```python
from build123d import *

# Parameters (mm, degrees)
BOSS_EXTRUDE1_DEPTH = 40
CUT_EXTRUDE1_REACH  = 53.556
SKETCH2_R           = 2.5
CUT_EXTRUDE2_REACH  = 53.556
SKETCH3_R           = 2.5
SKETCH4_W           = 70
SKETCH4_H           = 70
BOSS_EXTRUDE2_DEPTH = 3
SKETCH8_W           = 54
SKETCH8_H           = 54
SKETCH8_W_2         = 50
SKETCH8_H_2         = 50
CUT_EXTRUDE7_DEPTH  = 0.5
CUT_EXTRUDE8_REACH  = 112.467
SKETCH9_R           = 1.55
CUT_EXTRUDE9_REACH  = 112.467
SKETCH10_W          = 40
SKETCH10_H          = 20
FILLET1_R           = 5


with BuildPart() as part:
    # Sketch1 → Boss-Extrude1 (new body)
    with BuildSketch(Plane.XY):
        Polygon((0, 0), (0, 23), (23, 23), (23, 20), (3, 20), (3, 0), align=None)
    extrude(amount=BOSS_EXTRUDE1_DEPTH)

    # Sketch2 → Cut-Extrude1 (cut, up to next)
    with BuildSketch(Plane(origin=(0, 23, 0), x_dir=(1, 0, 0), z_dir=(0, 1, 0)), mode=Mode.PRIVATE) as cut_extrude1_sk1:
        with Locations(Location((13, -10, 0), (0, 0, 270))):
            Circle(SKETCH2_R)
    cut_extrude1_tool1 = extrude(cut_extrude1_sk1.sketch, amount=-CUT_EXTRUDE1_REACH, mode=Mode.PRIVATE) & part.part
    # Sketch2 → Cut-Extrude1 (cut, up to next)
    with BuildSketch(Plane(origin=(0, 23, 0), x_dir=(1, 0, 0), z_dir=(0, 1, 0)), mode=Mode.PRIVATE) as cut_extrude1_sk2:
        with Locations(Location((13, -30, 0), (0, 0, 270))):
            Circle(SKETCH2_R)
    cut_extrude1_tool2 = extrude(cut_extrude1_sk2.sketch, amount=-CUT_EXTRUDE1_REACH, mode=Mode.PRIVATE) & part.part
    add(cut_extrude1_tool1.solids().sort_by_distance((13, 23, 10))[0], mode=Mode.SUBTRACT)
    add(cut_extrude1_tool2.solids().sort_by_distance((13, 23, 30))[0], mode=Mode.SUBTRACT)

    # Sketch3 → Cut-Extrude2 (cut, up to next)
    with BuildSketch(Plane.ZY, mode=Mode.PRIVATE) as cut_extrude2_sk1:
        with Locations((10, 10)):
            Circle(SKETCH3_R)
    cut_extrude2_tool1 = extrude(cut_extrude2_sk1.sketch, amount=-CUT_EXTRUDE2_REACH, mode=Mode.PRIVATE) & part.part
    # Sketch3 → Cut-Extrude2 (cut, up to next)
    with BuildSketch(Plane.ZY, mode=Mode.PRIVATE) as cut_extrude2_sk2:
        with Locations((30, 10)):
            Circle(SKETCH3_R)
    cut_extrude2_tool2 = extrude(cut_extrude2_sk2.sketch, amount=-CUT_EXTRUDE2_REACH, mode=Mode.PRIVATE) & part.part
    add(cut_extrude2_tool1.solids().sort_by_distance((0, 10, 10))[0], mode=Mode.SUBTRACT)
    add(cut_extrude2_tool2.solids().sort_by_distance((0, 10, 30))[0], mode=Mode.SUBTRACT)

    # Sketch4 → Boss-Extrude2 (add)
    with BuildSketch(Plane(origin=(0, 23, 0), x_dir=(1, 0, 0), z_dir=(0, 1, 0))):
        with Locations((58, -20)):
            Rectangle(SKETCH4_W, SKETCH4_H)
    extrude(amount=-BOSS_EXTRUDE2_DEPTH)

    # Sketch8 → Cut-Extrude7 (cut)
    with BuildSketch(Plane(origin=(0, 23, 0), x_dir=(1, 0, 0), z_dir=(0, 1, 0))):
        with Locations((58, -20)):
            Rectangle(SKETCH8_W, SKETCH8_H)
        with Locations((58, -20)):
            Rectangle(SKETCH8_W_2, SKETCH8_H_2, mode=Mode.SUBTRACT)
    extrude(amount=-CUT_EXTRUDE7_DEPTH, mode=Mode.SUBTRACT)

    # Sketch9 → Cut-Extrude8 (cut, up to next)
    with BuildSketch(Plane(origin=(0, 23, 0), x_dir=(1, 0, 0), z_dir=(0, 1, 0)), mode=Mode.PRIVATE) as cut_extrude8_sk1:
        with Locations(Location((38, -40, 0), (0, 0, 270))):
            Circle(SKETCH9_R)
    cut_extrude8_tool1 = extrude(cut_extrude8_sk1.sketch, amount=-CUT_EXTRUDE8_REACH, mode=Mode.PRIVATE) & part.part
    # Sketch9 → Cut-Extrude8 (cut, up to next)
    with BuildSketch(Plane(origin=(0, 23, 0), x_dir=(1, 0, 0), z_dir=(0, 1, 0)), mode=Mode.PRIVATE) as cut_extrude8_sk2:
        with Locations(Location((38, 0, 0), (0, 0, 270))):
            Circle(SKETCH9_R)
    cut_extrude8_tool2 = extrude(cut_extrude8_sk2.sketch, amount=-CUT_EXTRUDE8_REACH, mode=Mode.PRIVATE) & part.part
    # Sketch9 → Cut-Extrude8 (cut, up to next)
    with BuildSketch(Plane(origin=(0, 23, 0), x_dir=(1, 0, 0), z_dir=(0, 1, 0)), mode=Mode.PRIVATE) as cut_extrude8_sk3:
        with Locations(Location((78, 0, 0), (0, 0, 270))):
            Circle(SKETCH9_R)
    cut_extrude8_tool3 = extrude(cut_extrude8_sk3.sketch, amount=-CUT_EXTRUDE8_REACH, mode=Mode.PRIVATE) & part.part
    # Sketch9 → Cut-Extrude8 (cut, up to next)
    with BuildSketch(Plane(origin=(0, 23, 0), x_dir=(1, 0, 0), z_dir=(0, 1, 0)), mode=Mode.PRIVATE) as cut_extrude8_sk4:
        with Locations(Location((78, -40, 0), (0, 0, 270))):
            Circle(SKETCH9_R)
    cut_extrude8_tool4 = extrude(cut_extrude8_sk4.sketch, amount=-CUT_EXTRUDE8_REACH, mode=Mode.PRIVATE) & part.part
    add(cut_extrude8_tool1.solids().sort_by_distance((38, 23, 40))[0], mode=Mode.SUBTRACT)
    add(cut_extrude8_tool2.solids().sort_by_distance((38, 23, 0))[0], mode=Mode.SUBTRACT)
    add(cut_extrude8_tool3.solids().sort_by_distance((78, 23, 0))[0], mode=Mode.SUBTRACT)
    add(cut_extrude8_tool4.solids().sort_by_distance((78, 23, 40))[0], mode=Mode.SUBTRACT)

    # Sketch10 → Cut-Extrude9 (cut, up to next)
    with BuildSketch(Plane.ZY, mode=Mode.PRIVATE) as cut_extrude9_sk1:
        with Locations((20, 10)):
            Rectangle(SKETCH10_W, SKETCH10_H)
    cut_extrude9_tool1 = extrude(cut_extrude9_sk1.sketch, amount=-CUT_EXTRUDE9_REACH, mode=Mode.PRIVATE) & part.part
    add(cut_extrude9_tool1.solids().sort_by_distance((0, 10, 20))[0], mode=Mode.SUBTRACT)

    # Fillet1
    fillet1_edges = [part.edges().sort_by_distance(p)[0] for p in [
        (23, 21.5, 40),
        (0, 21.5, 40),
        (23, 21.5, 55),
        (23, 21.5, -15),
        (93, 21.5, -15),
        (93, 21.5, 55),
        (0, 21.5, 0),
        (23, 21.5, 0),
    ]]
    fillet(fillet1_edges, radius=FILLET1_R)


solid = part.part
```
Input: part model. Units: mm. Frame: model coordinates. A direction names the side the tool comes from. Coordinates: 2 decimals unless noted, no trailing zeros. Loops run counter-clockwise (first coordinate to the right, second up) from the corner with the lowest first, then second, coordinate; pieces in that order, holes last. Notation, with made-up numbers: M 82.5,13 L 99.5,13 A9 ccw 99.5,20 Z; hole C 38,25.5 d5. An arc over 180 degrees is marked long. Answer in a Markdown table with one row per item.
1. Draft query along Z for faces 1 (the cylindrical face through (22, 21, -2)), 2 (the cylindrical face through (24, 21, 53)), 3 (the flat face through (93, 22, 20)), 4 (the cylindrical face through (79.537, 21.521, -0.202)). Return one class per face: pulls with the +Z half, pulls with the -Z half, needs draft (parallel to the pull), parting line crosses it, or undercut.
Response:
| item | result |
|---|---|
| face 1 | pulls with the -Z half |
| face 2 | pulls with the +Z half |
| face 3 | needs draft |
| face 4 | undercut |
2. Material intervals for line 1 (X direction, y = 22.75, z = 25.5); line 2 (Z direction, x = 78, y = 21.8); line 3 (Z direction, x = 42.5, y = 22.6), sorted ascending.
Response:
| item | result |
|---|---|
| line 1 | x = 0 to 31, 33 to 83, 85 to 93 |
| line 2 | z = -15 to -1.55, 1.55 to 38.45, 41.55 to 55 |
| line 3 | z = -15 to -7, -5 to 45, 47 to 55 |
3. Reachability of faces 5 (the flat face through (23, 22, 48)), 6 (the flat face through (12, 22, 0)), 7 (the cylindrical face through (36.487, 21.521, -0.336)) from +Z, -Z, +X, -X, +Y, -Y: full face, straight path, thin tool, end or side. Return the list, or none.
Response:
| item | result |
|---|---|
| face 5 | +Z, -X, +Y, -Y |
| face 6 | -Z, -X, +Y, -Y |
| face 7 | +Y, -Y |
4. Section A-A, the plane z = 30. Output: boundary loops of the cut face in (x, y).
Response:
| item | result |
|---|---|
| outline | M 0,20 L 10.5,20 L 10.5,23 L 0,23 Z; M 15.5,20 L 93,20 L 93,23 L 85,23 L 85,22.5 L 83,22.5 L 83,23 L 33,23 L 33,22.5 L 31,22.5 L 31,23 L 15.5,23 Z |
5. Section B-B, the plane x = 13. Output: boundary loops of the cut face in (y, z).
Response:
| item | result |
|---|---|
| outline | M 20,0 L 23,0 L 23,7.5 L 20,7.5 Z; M 20,12.5 L 23,12.5 L 23,27.5 L 20,27.5 Z; M 20,32.5 L 23,32.5 L 23,40 L 20,40 Z |
6. Section C-C, the plane y = 20.8. Output: boundary loops of the cut face in (x, z).
Response:
| item | result |
|---|---|
| outline | M 0,5 A5 ccw 5,0 L 18,0 A5 cw 23,-5 L 23,-10 A5 ccw 28,-15 L 88,-15 A5 ccw 93,-10 L 93,50 A5 ccw 88,55 L 28,55 A5 ccw 23,50 L 23,45 A5 cw 18,40 L 5,40 A5 ccw 0,35 Z; hole C 13,10 d5; hole C 13,30 d5; hole C 38,0 d3.1; hole C 38,40 d3.1; hole C 78,0 d3.1; hole C 78,40 d3.1 |
7. Section D-D, the plane x = 78. Output: boundary loops of the cut face in (y, z).
Response:
| item | result |
|---|---|
| outline | M 20,-15 L 23,-15 L 23,-7 L 22.5,-7 L 22.5,-5 L 23,-5 L 23,-1.55 L 20,-1.55 Z; M 20,1.55 L 23,1.55 L 23,38.45 L 20,38.45 Z; M 20,41.55 L 23,41.55 L 23,45 L 22.5,45 L 22.5,47 L 23,47 L 23,55 L 20,55 Z |
8. First-contact query: pin 1 (5 mm diameter, centred on x = 38, z = 0, fed in from +Y); pin 2 (0.9 mm diameter, centred on y = 22, z = 48, fed in from -X); pin 3 (1.9 mm diameter, centred on x = 78, z = 0, fed in from +Y). Flat tips, straight axial feed; report the tip coordinate or a pass-through.
Response:
| item | result |
|---|---|
| pin 1 | stops at y = 23 |
| pin 2 | stops at x = 23 |
| pin 3 | passes through |
